Build history of the part. All positions in model axes, mm. A direction names the side the tool comes from. Coordinates: 2 decimals unless noted, no trailing zeros. Loops run counter-clockwise (first coordinate to the right, second up) from the corner with the lowest first, then second, coordinate; pieces in that order, holes last.
Item 1: Cut at D-D (y = -4.25). List the corners of the cut face in (x, z), and give its area (3 significant figures).
Item 2: Cut at B-B (x = 3.5). List the corners of the cut face in (y, z), and give its area (3 significant figures).
Item 3: Cut at A-A (z = 5.1). List the corners of the cut face in (x, y), and give its area (3 significant figures).
Item 4: Mould opens along Y. For faces 3 (the face through (1, 5, 9)), 4 (the face through (2.586, 0.07, 6.533)), 5 (the face through (-4.4, 0.1, 8.9)) say: released by +Y, released by -Y, zero draft, split by the parting line, or undercut.
Item 5: 3-axis set-ups, long thin cutter, end or side, ignore diameter. For faces 1 (the face through (4.44, 2.86, 13.4)), 2 (the face through (-7.5, -1, 9)): which of +Z, -Z, +X, -X, +Y, -Y reach the whole face in a straight line?
Item 6: Cut at C-C (y = 0). List the corners of the cut face in (x, z).
Item 7: Drill centre lines: line 1 along Y through (x, z) = (-1.5, 6.25); line 2 along Z through (x, y) = (2, 0); line 3 along Z through (x, y) = (3.75, -0.5). Where is each one in solid material? Low to high.
Item 8: Flat gauge pin, fed straight in: pin 1 (5 mm diameter, centred on x = -1.5, y = 0, fed in from +Z). Where does the tip first touch, or does it go through?
from build123d import *

# Parameters (mm, degrees)
F0_R     = 2.9
F1_DEPTH = 18
F3_R     = 1.7
F4_DEPTH = 10.001
F2_R     = 3
F5_DEPTH = 8


with BuildPart() as f1:
    # F0 (on Top) → F1 (new body)
    with BuildSketch(Plane.XY):
        Polygon((7.5, -5), (7.5, 5), (-5.5, 5), (-7.5, 3), (-7.5, -5), align=None)
        with Locations((-1.5, 0)):
            Circle(F0_R, mode=Mode.SUBTRACT)
    extrude(amount=F1_DEPTH)

    # F3 (on face) → F4 (cut, through all)
    with BuildSketch(Plane(origin=(0, 5, 0), x_dir=(-1, 0, 0), z_dir=(0, 1, 0))):
        with Locations((-3.5, 5.1)):
            Circle(F3_R)
    extrude(amount=-F4_DEPTH, mode=Mode.SUBTRACT)

    # F2 (on face) → F5 (cut)
    with BuildSketch(Plane.YZ.offset(7.5)):
        with Locations((0, 12.5)):
            Circle(F2_R)
    extrude(amount=-F5_DEPTH, mode=Mode.SUBTRACT)


solid = f1.part
Filled sheet:
1. outline: (-7.5, 0) - (7.5, 0) - (7.5, 18) - (-7.5, 18) - close; hole circle Ø3.4 at (3.5, 5.1)
1. area: 261 mm2
2. outline: (-5, 0) - (5, 0) - (5, 3.4) - (-5, 3.4) - close; (-5, 6.8) - (5, 6.8) - (5, 18) - (-5, 18) - close; hole circle Ø6 at (0, 12.5)
2. area: 118 mm2
3. outline: (-7.5, -5) - (1.8, -5) - (1.8, 5) - (-5.5, 5) - (-7.5, 3) - close; (5.2, -5) - (7.5, -5) - (7.5, 5) - (5.2, 5) - close; hole circle Ø5.8 at (-1.5, 0)
3. area: 87.6 mm2
4. face 3: released by +Y
4. face 4: zero draft
4. face 5: undercut
5. face 1: +X
5. face 2: +Z, -Z, -X, +Y, -Y
6. outline: (-7.5, 0) - (-4.4, 0) - (-4.4, 18) - (-7.5, 18) - close; (1.4, 0) - (7.5, 0) - (7.5, 9.5) - (1.4, 9.5) - close; (1.4, 15.5) - (7.5, 15.5) - (7.5, 18) - (1.4, 18) - close; hole circle Ø3.4 at (3.5, 5.1)
7. line 1: y = -5 to -2.9, 2.9 to 5
7. line 2: z = 0 to 4.3, 5.9 to 9.5, 15.5 to 18
7. line 3: z = 0 to 3.42, 6.78 to 9.54, 15.46 to 18
8. pin 1: passes through
